```python
from build123d import *

# Parameters (mm, degrees)
SKETCH1_R           = 137.5
SKETCH1_R_2         = 12.5
SKETCH1_W           = 10
SKETCH1_H           = 3.175
SKETCH1_W_2         = 3.125
SKETCH1_H_2         = 6
BOSS_EXTRUDE1_DEPTH = 1.875


with BuildPart() as part:
    # Sketch1 → Boss-Extrude1 (new body, symmetric)
    with BuildSketch(Plane.XY):
        Circle(SKETCH1_R)
        Circle(SKETCH1_R_2, mode=Mode.SUBTRACT)
        with Locations((0, 66.5875)):
            Rectangle(SKETCH1_W, SKETCH1_H, mode=Mode.SUBTRACT)
        with Locations((-20, 66.5875)):
            Rectangle(SKETCH1_W, SKETCH1_H, mode=Mode.SUBTRACT)
        with Locations((20, 66.5875)):
            Rectangle(SKETCH1_W, SKETCH1_H, mode=Mode.SUBTRACT)
        with Locations((0, 48)):
            Rectangle(SKETCH1_W_2, SKETCH1_H_2, mode=Mode.SUBTRACT)
        Polygon((61.541281903, 29.757372981), (56.541281903, 38.417627019), (53.791651246, 36.830127019), (58.791651246, 28.169872981), align=None, mode=Mode.SUBTRACT)
        Polygon((51.541281903, 47.077881057), (46.541281903, 55.738135095), (43.791651246, 54.150635095), (48.791651246, 45.490381057), align=None, mode=Mode.SUBTRACT)
        Polygon((71.541281903, 12.436864905), (68.791651246, 10.849364905), (63.791651246, 19.509618943), (66.541281903, 21.097118943), align=None, mode=Mode.SUBTRACT)
        Polygon((44.948545593, 24.146835307), (43.386045593, 26.853164693), (38.18989317, 23.853164693), (39.75239317, 21.146835307), align=None, mode=Mode.SUBTRACT)
        Polygon((56.541281903, -38.417627019), (61.541281903, -29.757372981), (58.791651246, -28.169872981), (53.791651246, -36.830127019), align=None, mode=Mode.SUBTRACT)
        Polygon((66.541281903, -21.097118943), (71.541281903, -12.436864905), (68.791651246, -10.849364905), (63.791651246, -19.509618943), align=None, mode=Mode.SUBTRACT)
        Polygon((46.541281903, -55.738135095), (43.791651246, -54.150635095), (48.791651246, -45.490381057), (51.541281903, -47.077881057), align=None, mode=Mode.SUBTRACT)
        Polygon((43.386045593, -26.853164693), (44.948545593, -24.146835307), (39.75239317, -21.146835307), (38.18989317, -23.853164693), align=None, mode=Mode.SUBTRACT)
        with Locations((0, -66.5875)):
            Rectangle(SKETCH1_W, SKETCH1_H, mode=Mode.SUBTRACT)
        with Locations((20, -66.5875)):
            Rectangle(SKETCH1_W, SKETCH1_H, mode=Mode.SUBTRACT)
        with Locations((-20, -66.5875)):
            Rectangle(SKETCH1_W, SKETCH1_H, mode=Mode.SUBTRACT)
        with Locations((0, -48)):
            Rectangle(SKETCH1_W_2, SKETCH1_H_2, mode=Mode.SUBTRACT)
        Polygon((-61.541281903, -29.757372981), (-56.541281903, -38.417627019), (-53.791651246, -36.830127019), (-58.791651246, -28.169872981), align=None, mode=Mode.SUBTRACT)
        Polygon((-51.541281903, -47.077881057), (-46.541281903, -55.738135095), (-43.791651246, -54.150635095), (-48.791651246, -45.490381057), align=None, mode=Mode.SUBTRACT)
        Polygon((-71.541281903, -12.436864905), (-68.791651246, -10.849364905), (-63.791651246, -19.509618943), (-66.541281903, -21.097118943), align=None, mode=Mode.SUBTRACT)
        Polygon((-44.948545593, -24.146835307), (-43.386045593, -26.853164693), (-38.18989317, -23.853164693), (-39.75239317, -21.146835307), align=None, mode=Mode.SUBTRACT)
        Polygon((-56.541281903, 38.417627019), (-61.541281903, 29.757372981), (-58.791651246, 28.169872981), (-53.791651246, 36.830127019), align=None, mode=Mode.SUBTRACT)
        Polygon((-66.541281903, 21.097118943), (-71.541281903, 12.436864905), (-68.791651246, 10.849364905), (-63.791651246, 19.509618943), align=None, mode=Mode.SUBTRACT)
        Polygon((-46.541281903, 55.738135095), (-43.791651246, 54.150635095), (-48.791651246, 45.490381057), (-51.541281903, 47.077881057), align=None, mode=Mode.SUBTRACT)
        Polygon((-43.386045593, 26.853164693), (-44.948545593, 24.146835307), (-39.75239317, 21.146835307), (-38.18989317, 23.853164693), align=None, mode=Mode.SUBTRACT)
    extrude(amount=BOSS_EXTRUDE1_DEPTH, both=True)


solid = part.part
```
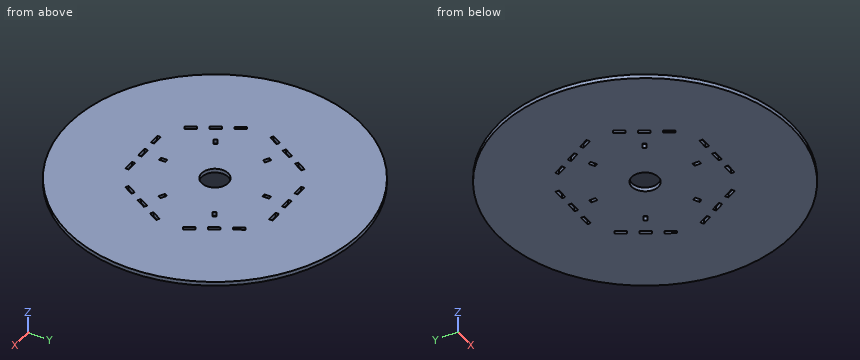
Here's how the part is built. I have some questions about the finished solid (model axes, mm). Give positions to 0.01 mm unless a question says otherwise; leave off trailing zeros. Loops run counter-clockwise (first coordinate to the right, second up) from the corner with the lowest first, then second, coordinate; pieces in that order, holes last. Notation, with made-up numbers: M -15.75,13 L 33.25,13 A12 ccw 33.25,29 Z; hole C -14.5,-35 d6. An arc over 180 degrees is marked long. Return JSON: item names as keys, results as strings.
Item 1: Imagine slicing it at D-D on y = -99. List the corners of the cut face in (x, z) for me (3 decimals).
A:
{"outline": "M -95.421,-1.875 L 95.421,-1.875 L 95.421,1.875 L -95.421,1.875 Z"}
Item 2: Imagine slicing it at B-B on z = -0.4. State how many separate pieces and enclosed holes the cut face has, then the cut area to 3 significant figures.
A:
{"separate pieces": "1", "enclosed holes": "25", "area": "58,200 mm^2"}
Item 3: Please list where these lines run through material, in increasing order: line 1 (Y direction, x = 0, z = -0.2) (3 decimals); line 2 (X direction, y = -23, z = -1.2); line 3 (Y direction, x = -59, z = 1.75).
A:
{"line 1": "y = -137.5 to -68.175, -65 to -51, -45 to -12.5, 12.5 to 45, 51 to 65, 68.175 to 137.5", "line 2": "x = -135.56 to -42.96, -38.68 to 38.68, 42.96 to 135.56", "line 3": "y = -124.2 to -34.16, -28.29 to 28.29, 34.16 to 124.2"}
Item 4: Imagine slicing it at A-A on y = 0. List the corners of the cut face in (x, z) for me (3 decimals).
A:
{"outline": "M -137.5,-1.875 L -12.5,-1.875 L -12.5,1.875 L -137.5,1.875 Z; M 12.5,-1.875 L 137.5,-1.875 L 137.5,1.875 L 12.5,1.875 Z"}
Item 5: Imagine slicing it at C-C on x = -104.5. List the corners of the cut face in (y, z) for me (3 decimals).
A:
{"outline": "M -89.364,-1.875 L 89.364,-1.875 L 89.364,1.875 L -89.364,1.875 Z"}
Item 6: I'm going to push flat-ended pins straight in: pin 1 Ø1.9 at (x, z) = (-22.5, 0.5) entering from -Y; pin 2 Ø1.1 at (x, z) = (18.5, -0.5) entering from -Y; pin 3 Ø1.6 at (y, z) = (67, 0) entering from +X. Where does each tip first touch, or does it pass through?
A:
{"pin 1": "stops at y = -135.8", "pin 2": "stops at y = -136.32", "pin 3": "stops at x = 120.51"}
